Model file for the job. Use its own axes, mm. Face numbers are marked on the shaded views. A direction names the side the tool comes from. Round coordinates to 2 decimals unless told otherwise and drop trailing zeros. Loops run counter-clockwise (first coordinate to the right, second up) from the corner with the lowest first, then second, coordinate; pieces in that order, holes last. Notation, with made-up numbers: (61, 23.25) - (70, 23.25) arc R9 cw to (70, 40.25) - close; hole circle Ø4 at (-2.75, 32). An arc over 180 degrees is marked (long way). Use one line per item in the form item = value.
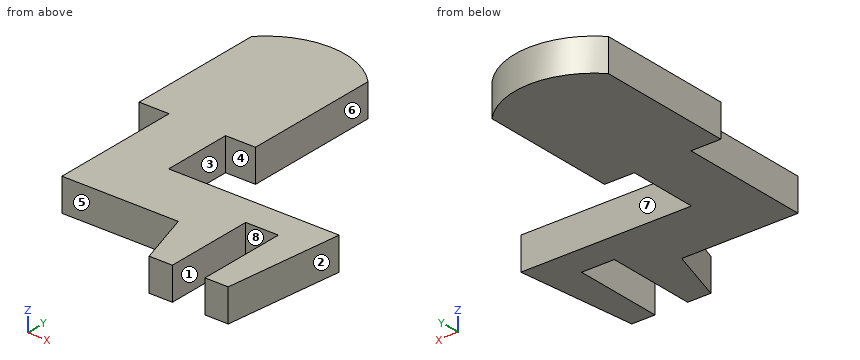
from build123d import *

# Parameters (mm, degrees)
BASE_EXTRUDE_DEPTH = 3


with BuildPart() as part:
    # Sketch1 → Base-Extrude (new body)
    with BuildSketch(Plane.XY):
        with BuildLine():
            Line((540.410759596, 46.36273023), (540.410759596, 39.95336404))
            Line((540.410759596, 39.95336404), (556.06264322, 39.95336404))
            Line((556.06264322, 39.95336404), (554.842233973, 28.969820695))
            Line((554.842233973, 28.969820695), (552.70789796, 28.969820695))
            Line((552.70789796, 28.969820695), (552.714937566, 37.219817691))
            Line((552.714937566, 37.219817691), (549.714937566, 37.219817691))
            Line((549.714937566, 37.219817691), (549.714937566, 28.969817691))
            Line((549.714937566, 28.969817691), (547.580602727, 28.972055819))
            Line((547.580602727, 28.972055819), (545.902566239, 34.311250108))
            Line((545.902566239, 34.311250108), (535.22410772, 34.311250108))
            Line((535.22410772, 34.311250108), (535.22410772, 46.36273023))
            Line((535.22410772, 46.36273023), (532.478204398, 46.36273023))
            Line((532.478204398, 46.36273023), (532.478204398, 46.515272643))
            Line((532.478204398, 46.515272643), (532.478204398, 59.024310063))
            ThreePointArc((532.478204398, 59.024310063), (537.817433658, 61.336415723), (543.156662918, 59.024310063))
            Line((543.156662918, 59.024310063), (543.156662918, 46.36273023))
            Line((543.156662918, 46.36273023), (540.410759596, 46.36273023))
        make_face()
    extrude(amount=BASE_EXTRUDE_DEPTH)


solid = part.part
1. Tool access for the marked faces 5, 6, 7 and 8: list every direction of +Z, -Z, +X, -X, +Y, -Y with a clear straight run to the whole face (end or side of a thin tool).
Geometry check:
face_5 = +Z, -Z, -X, -Y
face_6 = +Z, -Z, +X, +Y
face_7 = +Z, -Z, +X
face_8 = +Z, -Z, -Y
2. Cut at C-C, the plane x = 545.25. Give the cut face in (y, z).
Geometry check:
outline = (34.31, 0) - (39.95, 0) - (39.95, 3) - (34.31, 3) - close
3. Cut at D-D, the plane y = 57. Give the cut face in (x, z).
Geometry check:
outline = (532.48, 0) - (543.16, 0) - (543.16, 3) - (532.48, 3) - close
4. Pull direction Y, two halves, no side cores. Call the marked faces 1, 2, 3 and 4: +Y half, -Y half, draft (parallel to the pull), parting line (faces both ways), or undercut.
Geometry check:
face_1 = draft
face_2 = -Y half
face_3 = undercut
face_4 = undercut
5. Wall check: probe 1 along Y at (x, z) = (550.75, 2.4); probe 2 along Y at (x, z) = (540.75, 0.45); probe 3 along X at (y, z) = (55, 1.2). Give the ranges that are in metal, low to high.
Geometry check:
probe_1 = 37.22 to 39.95
probe_2 = 34.31 to 39.95, 46.36 to 60.72
probe_3 = 532.48 to 543.16
6. Cut at A-A, the plane y = 31. Give the cut face in (x, z).
Geometry check:
outline = (546.94, 0) - (549.71, 0) - (549.71, 3) - (546.94, 3) - close; (552.71, 0) - (555.07, 0) - (555.07, 3) - (552.71, 3) - close
7. Cut at B-B, the plane z = 1.15. Give the cut face in (x, y).
Geometry check:
outline = (532.48, 46.36) - (535.22, 46.36) - (535.22, 34.31) - (545.9, 34.31) - (547.58, 28.97) - (549.71, 28.97) - (549.71, 37.22) - (552.71, 37.22) - (552.71, 28.97) - (554.84, 28.97) - (556.06, 39.95) - (540.41, 39.95) - (540.41, 46.36) - (543.16, 46.36) - (543.16, 59.02) arc R7.32 ccw to (532.48, 59.02) - close
8. Flat gauge pins, fed straight in: pin 1 (1.4 mm diameter, centred on x = 533, z = 2, fed in from -Y); pin 2 (1.5 mm diameter, centred on y = 31.5, z = 1.5, fed in from +X); pin 3 (1.5 mm diameter, centred on y = 38.5, z = 1, fed in from -X). Where does each tip first touch, or does it go through?
Geometry check:
pin_1 = 46.36
pin_2 = 555.21
pin_3 = 535.22
